Input: part model. Units: mm. Frame: model coordinates. A direction names the side the tool comes from. Coordinates: 2 decimals unless noted, no trailing zeros. Order: outer loops, then holes, each group sorted by start corner. A loop starts at its lowest first (then second) coordinate and runs counter-clockwise, first axis right, second up. Notation, with made-up numbers: (74, 19.5) -> (102, 19.5) arc R25 ccw to (102, 46.5) -> close; hole circle Ø1 at (62, 71). An arc over 180 degrees is marked (long way). Write each question's results on one line, items separated by ' | '.
```python
from build123d import *

# Parameters (mm, degrees)
BOSS_EXTRUDE1_DEPTH = 10
SKETCH3_W           = 45
SKETCH3_H           = 3
BOSS_EXTRUDE2_DEPTH = 6.5
SKETCH4_R           = 3
CUT_EXTRUDE2_DEPTH  = 10
SKETCH5_R           = 2.5
BOSS_EXTRUDE3_DEPTH = 10


with BuildPart() as part:
    # Sketch2 → Boss-Extrude1 (new body)
    with BuildSketch(Plane.XY):
        Polygon((0, 0), (100, 0), (100, 12), (45, 52), (45, 100), (0, 100), align=None)
    extrude(amount=-BOSS_EXTRUDE1_DEPTH)

    # Sketch3 → Boss-Extrude2 (add)
    with BuildSketch(Plane.XY):
        with Locations((22.5, 98.5)):
            Rectangle(SKETCH3_W, SKETCH3_H)
        with Locations((22.5, 59.5)):
            Rectangle(SKETCH3_W, SKETCH3_H)
    extrude(amount=BOSS_EXTRUDE2_DEPTH)

    # Sketch4 → Cut-Extrude2 (cut)
    with BuildSketch(Plane.XY):
        with Locations((10, 79)):
            Circle(SKETCH4_R)
        with Locations((35, 79)):
            Circle(SKETCH4_R)
    extrude(amount=-CUT_EXTRUDE2_DEPTH, mode=Mode.SUBTRACT)

    # Sketch5 → Boss-Extrude3 (add)
    with BuildSketch(Plane.XY):
        with Locations((16.467286656, 7.268319627)):
            Circle(SKETCH5_R)
        with Locations((32.934573311, 14.536639255)):
            Circle(SKETCH5_R)
        with Locations((56.720654036, 25.035323161)):
            Circle(SKETCH5_R)
    extrude(amount=BOSS_EXTRUDE3_DEPTH)


solid = part.part
```
(1) Line query: line 1 along Y through (x, z) = (10, -4.5); line 2 along Z through (x, y) = (49.5, 38.5); line 3 along X through (y, z) = (91, -7.75). Output: solid intervals per line, ascending. Write a range as from..to.
Return value:
line 1: 0..76, 82..100 | line 2: -10..0 | line 3: 0..45
(2) Cut plane D-D, the plane z = -7.5. Return loops of the section in (x, y).
Return value:
outline: (0, 0) -> (100, 0) -> (100, 12) -> (45, 52) -> (45, 100) -> (0, 100) -> close; hole circle Ø6 at (10, 79); hole circle Ø6 at (35, 79)
(3) Pin query (flat end, axial travel): P1, Ø1.5, axis at x = 24.5, y = 59, coming from the +Z side; P2, Ø12, axis at x = 14, z = 6.5, coming from the -Y side; P3, Ø2, axis at x = 32.5, z = 4, coming from the -Y side. Return the tip coordinate at first contact, or that it passes through.
Return value:
P1: z = 6.5 | P2: y = 4.77 | P3: y = 12.04
(4) Reachability of faces 1 (the face through (45, 76, -4)), 2 (the face through (38, 23, 0)), 3 (the face through (22, 99, 6.5)), 4 (the face through (9.35, 76.07, -4.93)), 5 (the face through (22, 61, 3)) from +Z, -Z, +X, -X, +Y, -Y: full face, straight path, thin tool, end or side. Return the list, or none.
Return value:
face 1: +Z, -Z, +X, +Y | face 2: +Z | face 3: +Z, +X, -X, +Y | face 4: +Z, -Z | face 5: +Z, +X, -X
(5) Cut plane B-B, the plane x = 10. Return loops of the section in (y, z).
Return value:
outline: (0, -10) -> (76, -10) -> (76, 0) -> (61, 0) -> (61, 6.5) -> (58, 6.5) -> (58, 0) -> (0, 0) -> close; (82, -10) -> (100, -10) -> (100, 6.5) -> (97, 6.5) -> (97, 0) -> (82, 0) -> close
(6) Cut plane C-C, the plane z = 3.5. Return loops of the section in (x, y), plus the area to 3 significant figures.
Return value:
outline: (0, 58) -> (45, 58) -> (45, 61) -> (0, 61) -> close; (0, 97) -> (45, 97) -> (45, 100) -> (0, 100) -> close; circle Ø5 at (16.47, 7.27); circle Ø5 at (32.93, 14.54); circle Ø5 at (56.72, 25.04) | area: 329 mm2
(7) Mould query, pull axis X, two halves, no side actions, for faces 6 (the face through (72.885, 31.72, -4.93)), 7 (the face through (22, 58, 3)), 8 (the face through (32.6, 77.2, -4.9)), 9 (the face through (0, 49, -4)). Classes: +X half, -X half, draft (parallel to the pull), parting line (faces both ways), or undercut.
Return value:
face 6: +X half | face 7: draft | face 8: undercut | face 9: -X half
(8) Cut plane A-A, the plane y = 79. Return loops of the section in (x, z), plus the area to 3 significant figures.
Return value:
outline: (0, -10) -> (7, -10) -> (7, 0) -> (0, 0) -> close; (13, -10) -> (32, -10) -> (32, 0) -> (13, 0) -> close; (38, -10) -> (45, -10) -> (45, 0) -> (38, 0) -> close | area: 330 mm2
